from build123d import *

# Parameters (mm, degrees)
SKETCH1_W           = 20.4
SKETCH1_H           = 20.4
SKETCH1_W_2         = 16.4
SKETCH1_H_2         = 16.4
BOSS_EXTRUDE1_DEPTH = 35
SKETCH2_W           = 20.4
SKETCH2_H           = 20.4
SKETCH2_W_2         = 13.834702386
SKETCH2_H_2         = 14.497254018
BOSS_EXTRUDE2_DEPTH = 3
SKETCH3_R           = 1.4
SKETCH3_R_2         = 2.5
CUT_EXTRUDE1_DEPTH  = 42.775590959
FILLET1_R           = 1


with BuildPart() as part:
    # Sketch1 → Boss-Extrude1 (new body)
    with BuildSketch(Plane.XY):
        Rectangle(SKETCH1_W, SKETCH1_H)
        Rectangle(SKETCH1_W_2, SKETCH1_H_2, mode=Mode.SUBTRACT)
    extrude(amount=-BOSS_EXTRUDE1_DEPTH)

    # Sketch2 → Boss-Extrude2 (add)
    with BuildSketch(Plane.XY):
        Rectangle(SKETCH2_W, SKETCH2_H)
        Rectangle(SKETCH2_W_2, SKETCH2_H_2, mode=Mode.SUBTRACT)
    extrude(amount=BOSS_EXTRUDE2_DEPTH)

    # Sketch3 → Cut-Extrude1 (cut, through all)
    with BuildSketch(Plane(origin=(10.2, 0, 0), x_dir=(0, 0, -1), z_dir=(1, 0, 0))):
        with Locations((3, 0)):
            Circle(SKETCH3_R)
        with Locations((29, 0)):
            Circle(SKETCH3_R)
        with Locations((15, 0)):
            Circle(SKETCH3_R_2)
    extrude(amount=-CUT_EXTRUDE1_DEPTH, mode=Mode.SUBTRACT)

    # Fillet1
    fillet1_edges = [part.edges().sort_by_distance(p)[0] for p in [
        (8.2, 0, -35),
        (0, -8.2, -35),
        (-8.2, 0, -35),
        (0, 8.2, -35),
    ]]
    fillet(fillet1_edges, radius=FILLET1_R)


solid = part.part
Verification items for the finished model (mm, model axes). A direction names the side the tool comes from. Give positions to 0.01 mm unless a question says otherwise; leave off trailing zeros. Order: outer loops, then holes, each group sorted by start corner. A loop starts at its lowest first (then second) coordinate and runs counter-clockwise, first axis right, second up. Notation, with made-up numbers: M 59,88.25 L 63,88.25 A14 ccw 63,112.25 Z; hole C 84,51.25 d8. An arc over 180 degrees is marked long. Answer as a JSON object with one key per item and string values. Group by question number.
1) Cross-section at D-D (z = -15). Enter the section's corners in (x, y), then the cut area to 3 significant figures.
2) Cross-section at B-B (z = -23). Enter the section's corners in (x, y).
3) Mould release check, pull along Y, two halves, no side actions. Record for faces 1 (the face through (0, -10.2, -16)), 2 (the face through (6.917, 0, 1)), 3 (the face through (-1, -10, -35)): released by +Y, released by -Y, zero draft, split by the parting line, or undercut.
4) Depth check by flat-ended pin: pin 1 Ø6 at (x, y) = (-6.5, 2) entering from +Z; pin 2 Ø3 at (y, z) = (0, -15) entering from +X. Enter the tip coordinate at first touch or a pass-through.
5) Scan lines: line 1 along X through (y, z) = (-4, -23.5); line 2 along Z through (x, y) = (8, 0.5). Record each from-to range of solid material in increasing order. Write a range as [from, to].
6) Cross-section at A-A (y = -4.5). Enter the section's corners in (x, z), then the cut area to 3 significant figures.
7) Cross-section at C-C (x = -4.5). Enter the section's corners in (y, z).
8) Access from +Z, -Z, +X, -X, +Y, -Y to the whole of each face (thin tool, end or side, straight path). Record for faces 4 (the face through (-9, 0, 3)), 5 (the face through (-6.917, 0, 1)), 6 (the face through (0.129, 8.501, -34.715)).
Result sheet:
{
 "1": {"outline": "M -10.2,-10.2 L 10.2,-10.2 L 10.2,-2.5 L 8.2,-2.5 L 8.2,-8.2 L -8.2,-8.2 L -8.2,-2.5 L -10.2,-2.5 Z; M -10.2,2.5 L -8.2,2.5 L -8.2,8.2 L 8.2,8.2 L 8.2,2.5 L 10.2,2.5 L 10.2,10.2 L -10.2,10.2 Z", "area": "127 mm2"},
 "2": {"outline": "M -10.2,-10.2 L 10.2,-10.2 L 10.2,10.2 L -10.2,10.2 Z; hole M -8.2,-8.2 L 8.2,-8.2 L 8.2,8.2 L -8.2,8.2 Z"},
 "3": {"face 1": "released by -Y", "face 2": "undercut", "face 3": "zero draft"},
 "4": {"pin 1": "stops at z = 3", "pin 2": "passes through"},
 "5": {"line 1": "x = [-10.2, -8.2], [8.2, 10.2]", "line 2": "z = [0, 3]"},
 "6": {"outline": "M -10.2,-35 L -9.2,-35 A1 ccw -8.2,-34 L -8.2,0 L -6.92,0 L -6.92,3 L -10.2,3 Z; M 6.92,0 L 8.2,0 L 8.2,-34 A1 ccw 9.2,-35 L 10.2,-35 L 10.2,3 L 6.92,3 Z", "area": "159 mm2"},
 "7": {"outline": "M -10.2,-35 L -9.2,-35 A1 ccw -8.2,-34 L -8.2,0 L -7.25,0 L -7.25,3 L -10.2,3 Z; M 7.25,0 L 8.2,0 L 8.2,-34 A1 ccw 9.2,-35 L 10.2,-35 L 10.2,3 L 7.25,3 Z"},
 "8": {"face 4": "+Z, +X, -X, +Y, -Y", "face 5": "+Z, -Z", "face 6": "-Z"}
}
